Part model, mm, in its own coordinate system. Give positions to 0.01 mm unless a question says otherwise; leave off trailing zeros. Write each loop counter-clockwise with the first axis right and the second up, starting at its lowest first coordinate (ties: lowest second). Pieces come first, ordered by that corner, then holes.
```python
from build123d import *

# Parameters (mm, degrees)
SALIENTE_EXTRUIR1_DEPTH      = 2.4
CROQUIS2_W                   = 0.7
CROQUIS2_H                   = 0.7
SALIENTE_EXTRUIR2_DEPTH      = 6
SALIENTE_EXTRUIR3_DEPTH      = 3
SALIENTE_EXTRUIR3_DEPTH_BACK = 2
CROQUIS3_W                   = 0.7
CROQUIS3_H                   = 0.7


with BuildPart() as part:
    # Croquis1 → Saliente-Extruir1 (new body)
    with BuildSketch(Plane(origin=(0, 0, 0), x_dir=(1, 0, 0), z_dir=(0, 1, 0))):
        Polygon((-2.25, 1.25), (-0.25, 1.25), (0, 1), (0.25, 1.25), (2.25, 1.25), (2.5, 1), (2.5, -1), (2.25, -1.25), (0.25, -1.25), (0, -1), (-0.25, -1.25), (-2.25, -1.25), (-2.5, -1), (-2.5, 1), align=None)
    extrude(amount=SALIENTE_EXTRUIR1_DEPTH)

    # Croquis2 → Saliente-Extruir2 (add)
    with BuildSketch(Plane(origin=(0, 2.4, 0), x_dir=(1, 0, 0), z_dir=(0, 1, 0))):
        with Locations((-1.25, 0)):
            Rectangle(CROQUIS2_W, CROQUIS2_H)
        with Locations((1.25, 0)):
            Rectangle(CROQUIS2_W, CROQUIS2_H)
    extrude(amount=SALIENTE_EXTRUIR2_DEPTH)

    # Croquis3 → Saliente-Extruir3 (add, two sides: drawn at the far end of the back side and taken through both)
    with BuildSketch(Plane.XZ.offset(-SALIENTE_EXTRUIR3_DEPTH_BACK)):
        with Locations((-1.25, 0)):
            Rectangle(CROQUIS3_W, CROQUIS3_H)
        with Locations((1.25, 0)):
            Rectangle(CROQUIS3_W, CROQUIS3_H)
    extrude(amount=SALIENTE_EXTRUIR3_DEPTH + SALIENTE_EXTRUIR3_DEPTH_BACK)


solid = part.part
```
1) Saw through at A-A, the plane y = -1.75. Write the cut outline in (x, z).
Answers follow:
outline: (-1.6, -0.35) - (-0.9, -0.35) - (-0.9, 0.35) - (-1.6, 0.35) - close; (0.9, -0.35) - (1.6, -0.35) - (1.6, 0.35) - (0.9, 0.35) - close
2) Saw through at B-B, the plane z = 0. Write the cut outline in (x, y).
Answers follow:
outline: (-2.5, 0) - (-1.6, 0) - (-1.6, -3) - (-0.9, -3) - (-0.9, 0) - (0.9, 0) - (0.9, -3) - (1.6, -3) - (1.6, 0) - (2.5, 0) - (2.5, 2.4) - (1.6, 2.4) - (1.6, 8.4) - (0.9, 8.4) - (0.9, 2.4) - (-0.9, 2.4) - (-0.9, 8.4) - (-1.6, 8.4) - (-1.6, 2.4) - (-2.5, 2.4) - close
3) Saw through at C-C, the plane y = 0.5. Write the cut outline in (x, z).
Answers follow:
outline: (-2.5, -1) - (-2.25, -1.25) - (-0.25, -1.25) - (0, -1) - (0.25, -1.25) - (2.25, -1.25) - (2.5, -1) - (2.5, 1) - (2.25, 1.25) - (0.25, 1.25) - (0, 1) - (-0.25, 1.25) - (-2.25, 1.25) - (-2.5, 1) - close
4) Wall check: L1, parallel to X at y = 3, z = 0.3; L2, parallel to Y at x = -0.9, z = 0.45; L3, parallel to Z at x = 1.3, y = 8. Give the ranges that are in metal, low to high.
Answers follow:
L1: x = -1.6 to -0.9, 0.9 to 1.6
L2: y = 0 to 2.4
L3: z = -0.35 to 0.35
5) Pin check, flat tips, straight feed: pin 1 Ø0.8 at (y, z) = (-1, 0) entering from +X; pin 2 Ø3 at (x, y) = (1, 5.5) entering from -Z; pin 3 Ø0.8 at (y, z) = (-2, 0) entering from -X. Stop position of each tip, or through.
Answers follow:
pin 1: stops at x = 1.6
pin 2: stops at z = -0.35
pin 3: stops at x = -1.6
6) Saw through at D-D, the plane x = 0.45. Write the cut outline in (y, z).
Answers follow:
outline: (0, -1.25) - (2.4, -1.25) - (2.4, 1.25) - (0, 1.25) - close
7) Two-plate mould, pull along X, no slides. Class faces 1 (the face through (2.5, 1, 0)), 2 (the face through (0, 0, 0)), 3 (the face through (1, 1, 1.25)): +X half, -X half, draft (parallel to the pull), parting line (faces both ways), or undercut.
Answers follow:
face 1: +X half
face 2: undercut
face 3: draft
